```python
from build123d import *

# Parameters (mm, degrees)
SKETCH_1_W          = 12
SKETCH_1_H          = 10
EXTRUDE_1_DEPTH     = 19
SKETCH_2_OUTSIDE_W  = 18.92
SKETCH_2_OUTSIDE_H  = 16.92
SKETCH_2_OUTSIDE_R  = 6
CUT_EXTRUDE_1_DEPTH = 19
SKETCH_3_W          = 24
SKETCH_3_H          = 10
EXTRUDE_2_DEPTH     = 9
SKETCH_4_R          = 1.5
EXTRUDE_3_DEPTH     = 10
SKETCH_9_R          = 0.8
CUT_EXTRUDE_2_DEPTH = 3
SKETCH_10_W         = 0.3
SKETCH_10_H         = 1.5
EXTRUDE_5_DEPTH     = 2.5
SKETCH_12_R         = 0.3
CUT_EXTRUDE_3_DEPTH = 7.6


with BuildPart() as part:
    # 草图1 → 凸台-拉伸1 (new body)
    with BuildSketch(Plane.XY):
        with Locations((6, 5)):
            Rectangle(SKETCH_1_W, SKETCH_1_H)
    extrude(amount=EXTRUDE_1_DEPTH)

    # 草图2 outside → 切除-拉伸1 (cut)
    with BuildSketch(Plane.XY):
        with Locations((6, 5)):
            Rectangle(SKETCH_2_OUTSIDE_W, SKETCH_2_OUTSIDE_H)
        with Locations((6, 5)):
            Circle(SKETCH_2_OUTSIDE_R, mode=Mode.SUBTRACT)
    extrude(amount=CUT_EXTRUDE_1_DEPTH, mode=Mode.SUBTRACT)

    # 草图3 → 凸台-拉伸2 (add)
    with BuildSketch(Plane.XY):
        with Locations((12, 5)):
            Rectangle(SKETCH_3_W, SKETCH_3_H)
    extrude(amount=EXTRUDE_2_DEPTH)

    # 草图4 → 凸台-拉伸3 (add)
    with BuildSketch(Plane.XY.offset(9)):
        with Locations(Location((18, 5, 0), (0, 0, 180))):
            Circle(SKETCH_4_R)
    extrude(amount=EXTRUDE_3_DEPTH)

    # 草图9 → 切除-拉伸2 (cut)
    with BuildSketch(Plane.XY.offset(9)):
        with Locations((13.5, 5)):
            Circle(SKETCH_9_R)
        with Locations((22.5, 5)):
            Circle(SKETCH_9_R)
    extrude(amount=-CUT_EXTRUDE_2_DEPTH, mode=Mode.SUBTRACT)

    # 草图10 → 凸台-拉伸5 (add)
    with BuildSketch(Plane.XY.offset(19)):
        with Locations((2.35, 5)):
            Rectangle(SKETCH_10_W, SKETCH_10_H)
        with Locations((9.65, 5)):
            Rectangle(SKETCH_10_W, SKETCH_10_H)
    extrude(amount=EXTRUDE_5_DEPTH)

    # 草图12 → 切除-拉伸3 (cut)
    with BuildSketch(Plane.ZY.offset(-2.2)):
        with Locations(Location((20.75, 5, 0), (0, 0, 270))):
            Circle(SKETCH_12_R)
    extrude(amount=-CUT_EXTRUDE_3_DEPTH, mode=Mode.SUBTRACT)


solid = part.part
```
CAD build for the part. Positions are in the model's coordinates, mm. A direction names the side the tool comes from. Round coordinates to 2 decimals unless told otherwise and drop trailing zeros. Loops run counter-clockwise (first coordinate to the right, second up) from the corner with the lowest first, then second, coordinate; pieces in that order, holes last. Notation, with made-up numbers: M 51.5,52 L 70.5,52 A20 cw 70.5,74 Z; hole C 72.5,80.25 d9. An arc over 180 degrees is marked long. Return JSON: item names as keys, results as strings. Group by question number.
(1) Saw through at C-C, the plane y = 2. List the corners of the cut face in (x, z), and give its area (3 significant figures).
(2) Saw through at D-D, the plane z = 11.25. List the corners of the cut face in (x, y), and give its area (3 significant figures).
(3) Wall check: probe 1 along Y at (x, z) = (13.5, 7.8); probe 2 along Y at (x, z) = (9.75, 20.75); probe 3 along Z at (x, y) = (2.4, 5). Give the ranges that are in metal, low to high. Write a range as [from, to].
(4) Saw through at B-B, the plane x = 22.5. List the corners of the cut face in (y, z), and give its area (3 significant figures).
(5) Tool access for faces 1 (the cylindrical face through (12, 5, 14)), 2 (the flat face through (1, 9, 9)), 3 (the flat face through (2.5, 5, 20)): list every direction of +Z, -Z, +X, -X, +Y, -Y with a clear straight run to the whole face (end or side of a thin tool).
(6) Saw through at A-A, the plane z = 20. List the corners of the cut face in (x, y).
(7) Mould opens along X. For faces 4 (the flat face through (24, 5, 4)), 5 (the flat face through (22, 5, 6)), 6 (the flat face through (9, 10, 7)) say: +X half, -X half, draft (parallel to the pull), parting line (faces both ways), or undercut.
(8) Drop flat-ended pins along their axis: P1, Ø5, axis at y = 8, z = 18.5, coming from the +X side; P2, Ø0.8, axis at x = 1.5, y = 8.5, coming from the +Z side; P3, Ø1.8, axis at x = 22.5, y = 4.5, coming from the +Z side; P4, Ø1, axis at y = 4.5, z = 12.5, coming from the -X side. Give the stop position or say it passes through.
Answer list:
{
 "1": {"outline": "M 0,0 L 24,0 L 24,9 L 11.2,9 L 11.2,19 L 0.8,19 L 0.8,9 L 0,9 Z", "area": "320 mm2"},
 "2": {"outline": "M 2.68,0 L 9.32,0 A6 ccw 9.32,10 L 2.68,10 A6 ccw Z; C 18,5 d3", "area": "111 mm2"},
 "3": {"probe 1": "[0, 4.2], [5.8, 10]", "probe 2": "[4.25, 4.7], [5.3, 5.75]", "probe 3": "[0, 20.45], [21.05, 21.5]"},
 "4": {"outline": "M 0,0 L 10,0 L 10,9 L 5.8,9 L 5.8,6 L 4.2,6 L 4.2,9 L 0,9 Z", "area": "85.2 mm2"},
 "5": {"face 1": "+Z", "face 2": "+Z, -X, +Y", "face 3": "+Z, +Y, -Y"},
 "6": {"outline": "M 2.2,4.25 L 2.5,4.25 L 2.5,5.75 L 2.2,5.75 Z; M 9.5,4.25 L 9.8,4.25 L 9.8,5.75 L 9.5,5.75 Z"},
 "7": {"face 4": "+X half", "face 5": "undercut", "face 6": "draft"},
 "8": {"P1": "x = 19.41", "P2": "z = 19", "P3": "z = 9", "P4": "x = 0"}
}
